Can you work these out from the model? Positions are in its coordinate system, mm. A direction names the side the tool comes from. Give positions to 0.01 mm unless a question says otherwise; leave off trailing zeros. Order: outer loops, then holes, each group sorted by start corner. A loop starts at its lowest first (then second) coordinate and runs counter-clockwise, first axis right, second up. Notation, with made-up numbers: M 62,-20 L 111,-20 A30 cw 111,2 Z; hole C 12.5,50 d1. An arc over 180 degrees is marked long. Answer as a JSON object with one key per item and string values.
```python
from build123d import *

# Parameters (mm, degrees)
F1_DEPTH = 7.62
F2_R     = 10.16
F3_R     = 1.26999


# Not quite as in the source:
# - a fillet or chamfer is up to 0.001 mm smaller than in the source, because OpenCascade refuses the exact size


with BuildPart() as f1:
    # F0 (on Top) → F1 (new body)
    with BuildSketch(Plane.XY):
        with BuildLine():
            ThreePointArc((0, -6.985), (-5.1498821976, 4.7189976002), (6.9584199662, 0.6087828631))
            Line((6.9584199662, 0.6087828631), (9.4887544993, 0.8301584497))
            ThreePointArc((9.4887544993, 0.8301584497), (-6.0928284325, 7.3214115232), (-2.54, -9.1800885072))
            Line((-2.54, -9.1800885072), (-2.54, -22.0943992214))
            Line((-2.54, -22.0943992214), (-2.54, -24.6343992214))
            ThreePointArc((-2.54, -24.6343992214), (2.6098821976, -36.3383968216), (-9.4984199662, -32.2281820845))
            Line((-9.4984199662, -32.2281820845), (-12.0287544993, -32.4495576711))
            ThreePointArc((-12.0287544993, -32.4495576711), (3.5528284325, -38.9408107447), (0, -22.4393107142))
            Line((0, -22.4393107142), (0, -9.525))
            Line((0, -9.525), (0, -6.985))
        make_face()
    extrude(amount=F1_DEPTH)

    # F2
    f2_edges = [f1.edges().sort_by_distance(p)[0] for p in [
        (-2.54, -9.180089, 3.81),
        (0, -22.439311, 3.81),
    ]]
    fillet(f2_edges, radius=F2_R)

    # F3 (radius 1.27 in the source; OpenCascade refuses exactly that, so slightly less here)
    f3_edges = [f1.edges().sort_by_distance(p)[0] for p in [
        (6.95842, 0.608783, 3.81),
        (9.488754, 0.830158, 3.81),
        (-12.028754, -32.449558, 3.81),
        (-9.49842, -32.228182, 3.81),
        (-2.54, -24.634399, 3.81),
        (0, -6.985, 3.81),
    ]]
    fillet(f3_edges, radius=F3_R)


solid = f1.part
```
1) I need wall thicknesses on L1, parallel to Y at x = 3.5, z = 6.75; L2, parallel to Y at x = 1.75, z = 3.5; L3, parallel to X at y = 0, z = 3.5 (3 decimals). Which ranges of each line are inside material? Lowest first, please.
Results found:
{"L1": "y = -38.98 to -35.13, -28.11 to -24.25, 6.04 to 8.86", "L2": "y = -40.12 to -37.13, -26.11 to -22.28, 6.76 to 9.36", "L3": "x = -9.525 to -6.985"}
2) I want a section at B-B on y = 3. Write out the boundary of the cut face in (x, z), and give its area (3 significant figures).
Results found:
{"outline": "M -9.04,0 L -6.31,0 L -6.31,7.62 L -9.04,7.62 Z; M 6.31,0 L 9.04,0 L 9.04,7.62 L 6.31,7.62 Z", "area": "41.6 mm²"}
3) I want a section at A-A on x = -7.5. Write out the boundary of the cut face in (y, z).
Results found:
{"outline": "M -39.75,0 L -36.54,0 L -36.54,7.62 L -39.75,7.62 Z; M -5.87,0 L 5.87,0 L 5.87,7.62 L -5.87,7.62 Z"}
4) Thinking about a two-plate mould opening in X: for faces 4 (the face through (-9.806, -32.57, 3.863)), 5 (the face through (-11.579, -32.844, 3.863)), 6 (the face through (0, -12, 4)), which applies, pulls with the +X half, pulls with the -X half, needs draft (parallel to the pull), parting line crosses it, or undercut?
Results found:
{"face 4": "undercut", "face 5": "pulls with the -X half", "face 6": "pulls with the +X half"}
5) I'm going to push flat-ended pins straight in: pin 1 Ø4 at (y, z) = (-15.5, 6) entering from -X; pin 2 Ø3 at (y, z) = (-35.5, 1) entering from +X; pin 3 Ø2 at (x, z) = (-6.5, 6.5) entering from -Y. Where does each tip first touch, or does it pass through?
Results found:
{"pin 1": "stops at x = -2.66", "pin 2": "stops at x = 6.68", "pin 3": "stops at y = -40.67"}
6) I want a section at C-C on x = -3.5. Write out the boundary of the cut face in (y, z).
Results found:
{"outline": "M -41.1,0 L -38.54,0 L -38.54,7.62 L -41.1,7.62 Z; M -10.73,0 L -6.04,0 L -6.04,7.62 L -10.73,7.62 Z; M 6.04,0 L 8.86,0 L 8.86,7.62 L 6.04,7.62 Z"}
7) For faces 1 (the face through (0.97, -20.91, 3.86)), 2 (the face through (-3.511, -10.705, 3.863)), 3 (the face through (7.286, 0.936, 3.863)), which set-ups out of +Z, -Z, +X, -X, +Y, -Y let a thin tool reach every point of the face, with its end or its side?
Results found:
{"face 1": "+Z, -Z, +X", "face 2": "+Z, -Z, -X", "face 3": "+Z, -Z"}
